Work out the finished part from the listing and answer in its coordinate system (mm). Round coordinates to 2 decimals unless told otherwise and drop trailing zeros. Write each loop counter-clockwise with the first axis right and the second up, starting at its lowest first coordinate (ties: lowest second). Pieces come first, ordered by that corner, then holes.
1. Find section B-B (x = 0). Write down the section's boundary in (y, z).
2. Find section A-A (y = 6.5). Write down the section's boundary in (x, z), and give its area (3 significant figures).
3. Flat-ended cylindrical pins translate along their axes: pin 1 Ø0.5 at (x, z) = (12, -0.5) entering from +Y; pin 2 Ø1.1 at (x, z) = (12, 0.5) entering from +Y; pin 3 Ø0.5 at (x, z) = (27, -0.5) entering from -Y. Find the tip coordinate at first contact, or state that the pin passes through.
4. Straight lines are drawn through the part: probe 1 along X at (y, z) = (20.5, 0.75); probe 2 along Y at (x, z) = (-4.5, 0.7); probe 3 along X at (y, z) = (27, 0.35). For each, find the intervals that lie inside material, in ascending order.
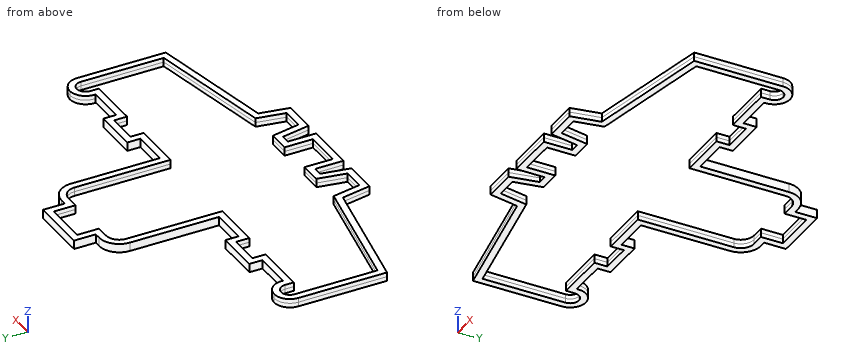
```python
from build123d import *

# Parameters (mm, degrees)
F1_DEPTH = 1


# Not quite as in the source:
# - a feature names something its author has since deleted; it is built from what else it names


with BuildPart() as f1:
    # F0 (on Top) → F1 (new body, symmetric)
    with BuildSketch(Plane.XY):
        with BuildLine():
            Line((6.5999999642, 31.0999999642), (0, 31.0999999642))
            Line((0, 31.0999999642), (-6.5999999642, 31.0999999642))
            Line((-6.5999999642, 31.0999999642), (-6.5999999642, 26.0999999642))
            Line((-6.5999999642, 26.0999999642), (-8, 26.0999999642))
            ThreePointArc((-8, 26.0999999642), (-11.2526911682, 24.7526911682), (-12.5999999642, 21.5))
            Line((-12.5999999642, 21.5), (-12.5999999642, 1.0999999642))
            Line((-12.5999999642, 1.0999999642), (-20.9000000358, 1.0999999642))
            Line((-20.9000000358, 1.0999999642), (-20.9000000358, 4.0999999642))
            Line((-20.9000000358, 4.0999999642), (-31.0999999642, 4.0999999642))
            Line((-31.0999999642, 4.0999999642), (-31.0999999642, 1.0999999642))
            Line((-31.0999999642, 1.0999999642), (-39.922291276, 1.0999999642))
            ThreePointArc((-39.922291276, 1.0999999642), (-40.8167184403, 3.8999999613), (-43.5, 5.0999999642))
            ThreePointArc((-43.5, 5.0999999642), (-46.045584387, 4.045584387), (-47.0999999642, 1.5))
            Line((-47.0999999642, 1.5), (-47.0999999642, -18.823789758))
            Line((-47.0999999642, -18.823789758), (-18.0247169235, -24.366737998))
            Line((-18.0247169235, -24.366737998), (-16.7816531759, -31.0999999642))
            Line((-16.7816531759, -31.0999999642), (-9.1183468241, -31.0999999642))
            Line((-9.1183468241, -31.0999999642), (-7.9183468241, -24.5999999642))
            Line((-7.9183468241, -24.5999999642), (-5.8499999642, -24.5999999642))
            Line((-5.8499999642, -24.5999999642), (-5.8499999642, -31.0999999642))
            Line((-5.8499999642, -31.0999999642), (0, -31.0999999642))
            Line((0, -31.0999999642), (5.8499999642, -31.0999999642))
            Line((5.8499999642, -31.0999999642), (5.8499999642, -24.5999999642))
            Line((5.8499999642, -24.5999999642), (7.9183468241, -24.5999999642))
            Line((7.9183468241, -24.5999999642), (9.1183468241, -31.0999999642))
            Line((9.1183468241, -31.0999999642), (16.7816531759, -31.0999999642))
            Line((16.7816531759, -31.0999999642), (18.0247169235, -24.366737998))
            Line((18.0247169235, -24.366737998), (47.0999999642, -18.823789758))
            Line((47.0999999642, -18.823789758), (47.0999999642, 1.5))
            ThreePointArc((47.0999999642, 1.5), (46.045584387, 4.045584387), (43.5, 5.0999999642))
            ThreePointArc((43.5, 5.0999999642), (40.8167184403, 3.8999999613), (39.922291276, 1.0999999642))
            Line((39.922291276, 1.0999999642), (31.0999999642, 1.0999999642))
            Line((31.0999999642, 1.0999999642), (31.0999999642, 4.0999999642))
            Line((31.0999999642, 4.0999999642), (20.9000000358, 4.0999999642))
            Line((20.9000000358, 4.0999999642), (20.9000000358, 1.0999999642))
            Line((20.9000000358, 1.0999999642), (12.5999999642, 1.0999999642))
            Line((12.5999999642, 1.0999999642), (12.5999999642, 21.5))
            ThreePointArc((12.5999999642, 21.5), (11.2526911682, 24.7526911682), (8, 26.0999999642))
            Line((8, 26.0999999642), (6.5999999642, 26.0999999642))
            Line((6.5999999642, 26.0999999642), (6.5999999642, 31.0999999642))
        make_face()
        with BuildLine():
            Line((-5, 29.5), (0, 29.5))
            Line((0, 29.5), (5, 29.5))
            Line((5, 29.5), (5, 24.5))
            Line((5, 24.5), (8, 24.5))
            ThreePointArc((8, 24.5), (10.1213203436, 23.6213203436), (11, 21.5))
            Line((11, 21.5), (11, -0.5))
            Line((11, -0.5), (22.5, -0.5))
            Line((22.5, -0.5), (22.5, 2.5))
            Line((22.5, 2.5), (29.5, 2.5))
            Line((29.5, 2.5), (29.5, -0.5))
            Line((29.5, -0.5), (41.5, -0.5))
            Line((41.5, -0.5), (41.5, 1.5))
            ThreePointArc((41.5, 1.5), (42.0857864376, 2.9142135624), (43.5, 3.5))
            ThreePointArc((43.5, 3.5), (44.9142135624, 2.9142135624), (45.5, 1.5))
            Line((45.5, 1.5), (45.5, -17.5))
            Line((45.5, -17.5), (16.65, -23))
            Line((16.65, -23), (15.45, -29.5))
            Line((15.45, -29.5), (10.45, -29.5))
            Line((10.45, -29.5), (9.25, -23))
            Line((9.25, -23), (4.25, -23))
            Line((4.25, -23), (4.25, -29.5))
            Line((4.25, -29.5), (0, -29.5))
            Line((0, -29.5), (-4.25, -29.5))
            Line((-4.25, -29.5), (-4.25, -23))
            Line((-4.25, -23), (-9.25, -23))
            Line((-9.25, -23), (-10.45, -29.5))
            Line((-10.45, -29.5), (-15.45, -29.5))
            Line((-15.45, -29.5), (-16.65, -23))
            Line((-16.65, -23), (-45.5, -17.5))
            Line((-45.5, -17.5), (-45.5, 1.5))
            ThreePointArc((-45.5, 1.5), (-44.9142135624, 2.9142135624), (-43.5, 3.5))
            ThreePointArc((-43.5, 3.5), (-42.0857864376, 2.9142135624), (-41.5, 1.5))
            Line((-41.5, 1.5), (-41.5, -0.5))
            Line((-41.5, -0.5), (-29.5, -0.5))
            Line((-29.5, -0.5), (-29.5, 2.5))
            Line((-29.5, 2.5), (-22.5, 2.5))
            Line((-22.5, 2.5), (-22.5, -0.5))
            Line((-22.5, -0.5), (-11, -0.5))
            Line((-11, -0.5), (-11, 21.5))
            ThreePointArc((-11, 21.5), (-10.1213203436, 23.6213203436), (-8, 24.5))
            Line((-8, 24.5), (-5, 24.5))
            Line((-5, 24.5), (-5, 29.5))
        make_face(mode=Mode.SUBTRACT)
    extrude(amount=F1_DEPTH, both=True)


solid = f1.part
```
Worked answers:
1. outline: (-31.1, -1) - (-29.5, -1) - (-29.5, 1) - (-31.1, 1) - close; (29.5, -1) - (31.1, -1) - (31.1, 1) - (29.5, 1) - close
2. outline: (-12.6, -1) - (-11, -1) - (-11, 1) - (-12.6, 1) - close; (11, -1) - (12.6, -1) - (12.6, 1) - (11, 1) - close
2. area: 6.40 mm2
3. pin 1: stops at y = 24.16
3. pin 2: stops at y = 24.54
3. pin 3: stops at y = -22.7
4. probe 1: x = -12.6 to -11, 11 to 12.6
4. probe 2: y = -31.1 to -23, 29.5 to 31.1
4. probe 3: x = -6.6 to -5, 5 to 6.6
